Autodesk Inventor part; units mm, degrees
ref_plane "YZ Plane" through (0, 0, 0) normal (1, 0, 0) x (0, 1, 0)
ref_plane "XZ Plane" through (0, 0, 0) normal (0, 1, 0) x (-1, 0, 0)
ref_plane "XY Plane" through (0, 0, 0) normal (0, 0, 1) x (1, 0, 0)
sketch "Esboço1" plane through (0, 0, 0) normal (0, 0, 1) x (1, 0, 0)
  line L0 (0, 0) -> (0, 17.5)
  arc A0 (0, 17.5) -> (-3, 20.5) centre (-3, 17.5) ccw
  line L1 (-3, 20.5) -> (-8, 20.5)
  arc A1 (-8, 20.5) -> (-9.5571, 19.7552) centre (-8, 18.5) ccw
  line L2 (-23.75, 1.5) -> (-14, 1.5)
  line L3 (-14, 1.5) -> (-14, 0)
  arc A2 (-23.9446, 1.9069) -> (-23.75, 1.5) centre (-23.75, 1.75) ccw
  line L4 (-23.9446, 1.9069) -> (-9.5571, 19.7552)
  line L5 (0, 0) -> (0, -17.5)
  arc A3 (-3, -20.5) -> (0, -17.5) centre (-3, -17.5) ccw
  line L6 (-3, -20.5) -> (-8, -20.5)
  arc A4 (-9.5571, -19.7552) -> (-8, -20.5) centre (-8, -18.5) ccw
  line L7 (-23.75, -1.5) -> (-14, -1.5)
  line L8 (-14, -1.5) -> (-14, 0)
  arc A5 (-23.75, -1.5) -> (-23.9446, -1.9069) centre (-23.75, -1.75) ccw
  line L9 (-23.9446, -1.9069) -> (-9.5571, -19.7552)
  point P0 (-7, 0)
  point P1 (-5.5, 20.5)
  point P2 (-5.5, -20.5)
extrude "Extrusão1" add sketch "Esboço1" along normal blind 3
properties part number "LEME"
Input: part model. Units: mm. Frame: model coordinates. A direction names the side the tool comes from. Give positions to 0.01 mm unless a question says otherwise; leave off trailing zeros. Loops run counter-clockwise (first coordinate to the right, second up) from the corner with the lowest first, then second, coordinate; pieces in that order, holes last. Notation, with made-up numbers: M 4.5,37.5 L 35.5,37.5 A17 ccw 35.5,70.5 Z; hole C -8,5 d9. An arc over 180 degrees is marked long. Use one line per item in the form item = value.
1. Line query: L1, parallel to X at y = 0, z = 2.75; L2, parallel to Y at x = -14.5, z = 0.4; L3, parallel to Y at x = -23, z = 0.55. Output: solid intervals per line, ascending.
Numbers:
L1 = -14 to 0
L2 = -13.62 to -1.5, 1.5 to 13.62
L3 = -3.08 to -1.5, 1.5 to 3.08
2. Reachability of faces 1 (the face through (-19, -1.5, 1)), 2 (the face through (-10, 0, 3)) from +Z, -Z, +X, -X, +Y, -Y: full face, straight path, thin tool, end or side. Return the list, or none.
Numbers:
face_1 = +Z, -Z, -X
face_2 = +Z, +X, -X, +Y, -Y
3. Section query A-A, the plane x = -16.75. Return the cut outline in (y, z).
Numbers:
outline = M -10.83,0 L -1.5,0 L -1.5,3 L -10.83,3 Z; M 1.5,0 L 10.83,0 L 10.83,3 L 1.5,3 Z
4. Section query D-D, the plane x = -20.5. Return the cut outline in (y, z), and give its area (3 significant figures).
Numbers:
outline = M -6.18,0 L -1.5,0 L -1.5,3 L -6.18,3 Z; M 1.5,0 L 6.18,0 L 6.18,3 L 1.5,3 Z
area = 28.1 mm²
5. Section query B-B, the plane z = 0.95. Return the cut outline in (x, y), and give its area (3 significant figures).
Numbers:
outline = M -23.94,-1.91 L -9.56,-19.76 A2 ccw -8,-20.5 L -3,-20.5 A3 ccw 0,-17.5 L 0,17.5 A3 ccw -3,20.5 L -8,20.5 A2 ccw -9.56,19.76 L -23.94,1.91 A0.25 ccw -23.75,1.5 L -14,1.5 L -14,-1.5 L -23.75,-1.5 A0.25 ccw Z
area = 669 mm²
6. Section query C-C, the plane y = 1. Return the cut outline in (x, z).
Numbers:
outline = M -14,0 L 0,0 L 0,3 L -14,3 Z
7. First-contact query: pin 1 (1.5 mm diameter, centred on x = -18.5, z = 1.5, fed in from +Y); pin 2 (1 mm diameter, centred on x = -13.5, z = 1.5, fed in from +Y). Flat tips, straight axial feed; report the tip coordinate or a pass-through.
Numbers:
pin_1 = 9.59
pin_2 = 15.48
